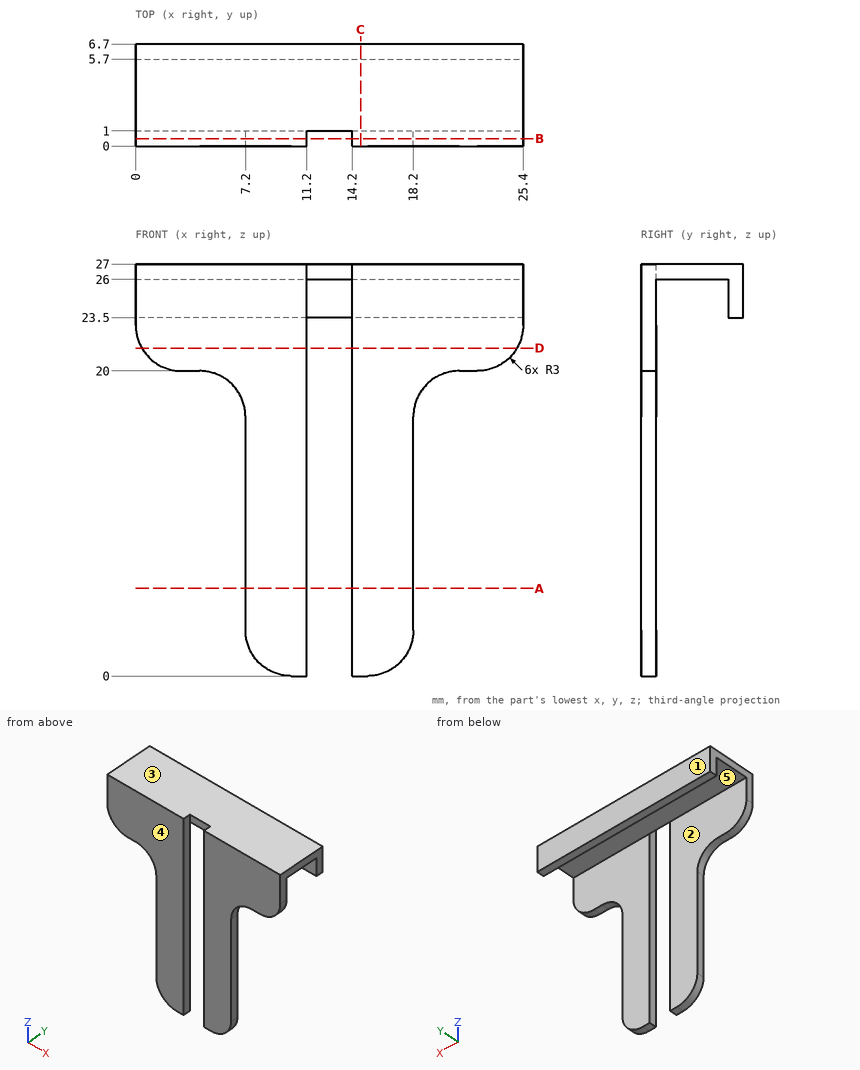
Could you check a few things on this drawing? It's one solid part, dimensions in mm from its lowest x, y, z. A direction names the side the tool comes from. Give positions to 0.01 mm unless a question says otherwise; leave off trailing zeros. Loops run counter-clockwise (first coordinate to the right, second up) from the corner with the lowest first, then second, coordinate; pieces in that order, holes last. Notation, with made-up numbers: (31, -13.75) -> (77, -13.75) arc R22 cw to (77, 14.25) -> close; hole circle Ø4 at (47, -19.75). An arc over 180 degrees is marked (long way). Use one line per item in the form item = value. Start each with the question number.
1) Please list where these lines run through material, in increasing order: line 1 along X through (y, z) = (0.75, 16.5); line 2 along Z through (x, y) = (7.5, 4); line 3 along Y through (x, z) = (10.75, 12.75).
2) Imagine slicing it at C-C (x = 14.75). Please give me the cut outline in (y, z), then the cut area to 3 significant figures.
3) Imagine slicing it at A-A (z = 5.75). Please give me the cut outline in (x, y).
4) Which directions (+Z, -Z, +X, -X, +Y, -Y) give clear straight access to the entire face, cutting with the end or side of a thin tool? Please do the marked faces 1 and 2.
5) Imagine slicing it at B-B (y = 0.5). Please give me the cut outline in (x, z), then the cut area to 3 significant figures.
6) Thinking about a two-plate mould opening in Y: for the marked faces 3, 4 and 5, which applies, +Y half, -Y half, draft (parallel to the pull), parting line (faces both ways), or undercut?
7) For P1, Ø1.4, axis at x = 11.5, y = 3, coming from the -Z side; P2, Ø0.8, axis at y = 0.5, z = 13, coming from the -X side; P3, Ø1.1, axis at x = 10.5, y = 6, coming from the -Z side; P4, Ø5, axis at x = 20.5, z = 14, coming from the -Y side, each with a flat end and sliding along its axis, tell me the tip position at first contact or that it passes through.
8) Imagine slicing it at D-D (z = 21.5). Please give me the cut outline in (x, y), then the cut area to 3 significant figures.
Check values:
q1.line_1 = 7.2 to 11.2, 14.2 to 18.2
q1.line_2 = 26 to 27
q1.line_3 = 0 to 1
q2.outline = (0, 0) -> (1, 0) -> (1, 26) -> (5.7, 26) -> (5.7, 23.5) -> (6.7, 23.5) -> (6.7, 27) -> (0, 27) -> close
q2.area = 35.2 mm^2
q3.outline = (7.2, 0) -> (11.2, 0) -> (11.2, 1) -> (7.2, 1) -> close; (14.2, 0) -> (18.2, 0) -> (18.2, 1) -> (14.2, 1) -> close
q4.face_1 = +Z, -Z, +X, -X, +Y
q4.face_2 = -Z, +X, -X
q5.outline = (0, 23) arc R3 ccw to (3, 20) -> (4.2, 20) arc R3 cw to (7.2, 17) -> (7.2, 3) arc R3 ccw to (10.2, 0) -> (11.2, 0) -> (11.2, 27) -> (0, 27) -> close; (14.2, 0) -> (15.2, 0) arc R3 ccw to (18.2, 3) -> (18.2, 17) arc R3 cw to (21.2, 20) -> (22.4, 20) arc R3 ccw to (25.4, 23) -> (25.4, 27) -> (14.2, 27) -> close
q5.area = 313 mm^2
q6.face_3 = draft
q6.face_4 = -Y half
q6.face_5 = undercut
q7.P1 = 26
q7.P2 = 7.2
q7.P3 = 23.5
q7.P4 = 0
q8.outline = (0.4, 0) -> (11.2, 0) -> (11.2, 1) -> (0.4, 1) -> close; (14.2, 0) -> (25, 0) -> (25, 1) -> (14.2, 1) -> close
q8.area = 21.6 mm^2
